Verification items for the finished model (mm, model axes). Round coordinates to 2 decimals unless told otherwise and drop trailing zeros. Loops run counter-clockwise (first coordinate to the right, second up) from the corner with the lowest first, then second, coordinate; pieces in that order, holes last. Notation, with made-up numbers: M -22.75,29 L 34.25,29 A24 ccw 34.25,47 Z; hole C 60.25,-0.75 d7. An arc over 180 degrees is marked long. One line per item, written item: value.
from build123d import *

# Parameters (mm, degrees)
EXTRUDE1_DEPTH = 292.1


with BuildPart() as part:
    # Sketch1 → Extrude1 (new body, symmetric)
    with BuildSketch(Plane.XY):
        with BuildLine():
            Line((1219.2, 19.05), (1219.2, 36.5125))
            ThreePointArc((1219.2, 36.5125), (1218.735032015, 37.635032015), (1217.6125, 38.1))
            Line((1217.6125, 38.1), (1185.2275, 38.1))
            Line((1185.2275, 38.1), (1185.2275, 39.6875))
            Line((1185.2275, 39.6875), (1217.6125, 39.6875))
            ThreePointArc((1217.6125, 39.6875), (1218.735032015, 40.152467985), (1219.2, 41.275))
            Line((1219.2, 41.275), (1219.2, 48.387))
            ThreePointArc((1219.2, 48.387), (1218.735032015, 49.509532015), (1217.6125, 49.9745))
            Line((1217.6125, 49.9745), (1199.5785, 49.9745))
            Line((1199.5785, 49.9745), (1199.5785, 51.562))
            Line((1199.5785, 51.562), (1217.6125, 51.562))
            ThreePointArc((1217.6125, 51.562), (1219.85756403, 50.63206403), (1220.7875, 48.387))
            Line((1220.7875, 48.387), (1220.7875, 19.05))
            Line((1220.7875, 19.05), (1219.2, 19.05))
        make_face()
    extrude(amount=EXTRUDE1_DEPTH, both=True)


solid = part.part
(1) Sectioned sample at A-A on x = 1211. Enter the section's corners in (y, z).
Completed:
outline: M 38.1,-292.1 L 39.69,-292.1 L 39.69,292.1 L 38.1,292.1 Z; M 49.97,-292.1 L 51.56,-292.1 L 51.56,292.1 L 49.97,292.1 Z
(2) Mould release check, pull along Y, two halves, no side actions. Record for faces 1 (the face through (1219.2, 28, 4)), 2 (the face through (1202, 38.1, 4)), 3 (the face through (1201, 39.688, 4)), 4 (the face through (1209, 49.974, 4)): +Y half, -Y half, draft (parallel to the pull), parting line (faces both ways), or undercut.
Completed:
face 1: draft
face 2: -Y half
face 3: undercut
face 4: undercut
(3) Sectioned sample at C-C on y = 28. Enter the section's corners in (x, z), and give its area (3 significant figures).
Completed:
outline: M 1219.2,-292.1 L 1220.79,-292.1 L 1220.79,292.1 L 1219.2,292.1 Z
area: 927 mm^2
(4) Depth check by flat-ended pin: pin 1 Ø6 at (y, z) = (37.5, 76) entering from -X; pin 2 Ø1.7 at (y, z) = (51, 106) entering from -X; pin 3 Ø2 at (y, z) = (44.5, 2) entering from -X; pin 4 Ø9.5 at (x, z) = (1200, 132.5) entering from -Y. Enter the tip coordinate at first touch or a pass-through.
Completed:
pin 1: stops at x = 1185.23
pin 2: stops at x = 1199.58
pin 3: stops at x = 1219.2
pin 4: stops at y = 38.1
(5) Thickness scan on L1, parallel to Y at x = 1208.5, z = -74; L2, parallel to Y at x = 1199, z = 85.5; L3, parallel to X at y = 45.5, z = 44.5. Record the ranges inside material, lowest first. Write a range as from..to.
Completed:
L1: y = 38.1..39.69, 49.97..51.56
L2: y = 38.1..39.69
L3: x = 1219.2..1220.79
